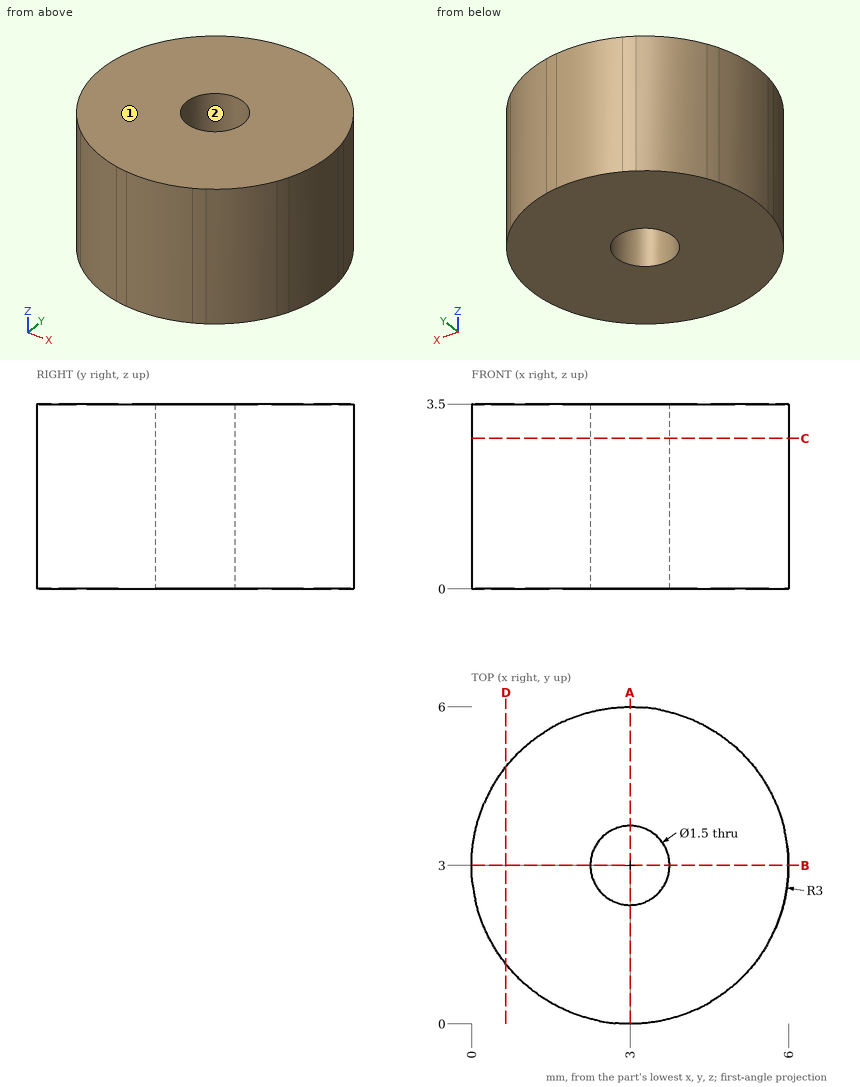
Geometry check sheet. Reference: drawing and pictorial views, mm from the part's lowest x, y, z. Round coordinates to 2 decimals unless told otherwise and drop trailing zeros. Order: outer loops, then holes, each group sorted by start corner. A loop starts at its lowest first (then second) coordinate and runs counter-clockwise, first axis right, second up. Notation, with made-up numbers: (12.5, -7) - (64.5, -7) arc R16 cw to (64.5, 1) - close; hole circle Ø6 at (70.5, 41). An arc over 180 degrees is marked (long way). One line per question, with ' | ' between items. Start each with the question number.
(1) Sectioned sample at D-D on x = 0.65. Record the cut outline in (y, z).
(2) Sectioned sample at C-C on z = 2.85. Record the cut outline in (x, y).
(3) Sectioned sample at A-A on x = 3. Record the cut outline in (y, z), and give its area (4 significant figures).
(4) Depth check by flat-ended pin: pin 1 Ø1 at (x, y) = (5, 4.5) entering from -Z; pin 2 Ø2 at (x, z) = (4.5, 1) entering from -Y. Enter the tip coordinate at first touch or a pass-through.
(5) Thickness scan on L1, parallel to Y at x = 3, z = 1.6; L2, parallel to X at y = 3.65, z = 0.6; L3, parallel to Y at x = 5.25, z = 2.55. Record the ranges inside material, lowest first. Write a range as [from, to].
(6) Release check for a two-part mould opening along Y. For the marked faces 1 and 2 record: released by +Y, released by -Y, zero draft, split by the parting line, or undercut.
Conclusion:
1) outline: (1.14, 0) - (4.86, 0) - (4.86, 3.5) - (1.14, 3.5) - close
2) outline: circle Ø6 at (3, 3); hole circle Ø1.5 at (3, 3)
3) outline: (0, 0) - (2.25, 0) - (2.25, 3.5) - (0, 3.5) - close; (3.75, 0) - (6, 0) - (6, 3.5) - (3.75, 3.5) - close | area: 15.75 mm2
4) pin 1: stops at z = 0 | pin 2: stops at y = 0.04
5) L1: y = [0, 2.25], [3.75, 6] | L2: x = [0.07, 2.63], [3.37, 5.93] | L3: y = [1.02, 4.98]
6) face 1: zero draft | face 2: undercut
